```python
from build123d import *

# Parameters (mm, degrees)
BOSS_EXTRUDE2_DEPTH = 18
SKETCH3_R           = 1.6
CUT_EXTRUDE1_DEPTH  = 24
CHAMFER1_SIZE       = 1.2


with BuildPart() as part:
    # Sketch2 → Boss-Extrude2 (new body)
    with BuildSketch(Plane.XY):
        Polygon((-3.1, 0), (3.1, 0), (3.1, -1.2), (10, -1.2), (10, -7.8), (4.9, -7.8), (4.9, -2.8), (-4.9, -2.8), (-4.9, -7.8), (-10, -7.8), (-10, -1.2), (-3.1, -1.2), align=None)
    extrude(amount=BOSS_EXTRUDE2_DEPTH)

    # Sketch3 → Cut-Extrude1 (cut)
    with BuildSketch(Plane(origin=(0, 0, 0), x_dir=(1, 0, 0), z_dir=(0, 1, 0))):
        with Locations(Location((0, -6, 0), (0, 0, 270))):
            Circle(SKETCH3_R)
    extrude(amount=-CUT_EXTRUDE1_DEPTH, mode=Mode.SUBTRACT)

    # Chamfer1
    chamfer1_edges = [part.edges().sort_by_distance(p)[0] for p in [
        (3.1, -1.2, 9),
        (-3.1, -1.2, 9),
    ]]
    chamfer(chamfer1_edges, length=CHAMFER1_SIZE - 0.0001)  # a hair under: the kernel refuses the full size


solid = part.part
```
Geometry: final body of the model. Coordinates: model frame, mm. A direction names the side the tool comes from. Round coordinates to 2 decimals unless told otherwise and drop trailing zeros. Order: outer loops, then holes, each group sorted by start corner. A loop starts at its lowest first (then second) coordinate and runs counter-clockwise, first axis right, second up. Notation, with made-up numbers: (35, -24) - (84, -24) arc R32 ccw to (84, 4) - close; hole circle Ø7 at (-14.5, 11). An arc over 180 degrees is marked (long way). Use CSV: the item, a comma, the result in double quotes. Start each with the question number.
Q1. Section query C-C (x = 0). Return loops of the section in (y, z).
Q2. Access query for faces 4 (the face through (4.9, -5, 9)), 5 (the face through (-7, -1.2, 9)), 6 (the face through (7, -1.2, 9)). Directions: +Z, -Z, +X, -X, +Y, -Y. A direction counts if a zero-diameter tool reaches every point of the face in a straight line with its end or side. Return the directions, or none.
Q3. First-contact query: pin 1 (6.5 mm diameter, centred on x = 8.5, z = 12.5, fed in from +Y); pin 2 (3 mm diameter, centred on x = 2.5, z = 5, fed in from -Y); pin 3 (1.5 mm diameter, centred on x = -2, y = -5.5, fed in from -Z); pin 4 (6.5 mm diameter, centred on x = -7, z = 4.5, fed in from +Y). Flat tips, straight axial feed; report the tip coordinate or a pass-through.
Q4. Section query B-B (y = -6.75). Return loops of the section in (x, z), and give its area (3 significant figures).
Q5. Material intervals for line 1 along X through (y, z) = (-4.75, 9); line 2 along X through (y, z) = (-1.5, 6); line 3 along Y through (x, z) = (7.5, 10), sorted ascending. Write a range as from..to.
Q6. Mould query, pull axis Z, two halves, no side actions, for faces 1 (the face through (0.481, -1.38, 7.526)), 2 (the face through (0, -2, 18)), 3 (the face through (3.7, -0.6, 8.9)). Classes: +Z half, -Z half, draft (parallel to the pull), parting line (faces both ways), or undercut.
Q7. Section query D-D (y = -2.5). Return loops of the section in (x, z).
Result set:
1,outline,"(-2.8, 0) - (0, 0) - (0, 4.4) - (-2.8, 4.4) - close; (-2.8, 7.6) - (0, 7.6) - (0, 18) - (-2.8, 18) - close"
2,face 4,"+Z, -Z, -Y"
2,face 5,"+Z, -Z, -X, +Y"
2,face 6,"+Z, -Z, +X, +Y"
3,pin 1,"stops at y = -1.2"
3,pin 2,"stops at y = -2.8"
3,pin 3,"passes through"
3,pin 4,"stops at y = -0.65"
4,outline,"(-10, 0) - (-4.9, 0) - (-4.9, 18) - (-10, 18) - close; (4.9, 0) - (10, 0) - (10, 18) - (4.9, 18) - close"
4,area,"184 mm2"
5,line 1,"x = -10..-4.9, 4.9..10"
5,line 2,"x = -10..-1.6, 1.6..10"
5,line 3,"y = -7.8..-1.2"
6,face 1,"undercut"
6,face 2,"+Z half"
6,face 3,"draft"
7,outline,"(-10, 0) - (10, 0) - (10, 18) - (-10, 18) - close; hole circle Ø3.2 at (0, 6)"
